```python
from build123d import *

# Parameters (mm, degrees)
F1_W     = 25.4
F1_H     = 12.7
F2_DEPTH = 25.4
F0_W     = 38.1
F0_H     = 50.8
F3_DEPTH = 12.7
F4_R     = 10.3422808599
F5_DEPTH = 12.701
F6_R     = 19.04999
F7_W     = 12.7
F7_H     = 6.35
F8_DEPTH = 12.7


# Not quite as in the source:
# - a fillet or chamfer is up to 0.001 mm smaller than in the source, because OpenCascade refuses the exact size


with BuildPart() as f2:
    # F1 (on face) → F2 (new body)
    with BuildSketch(Plane.XY):
        with Locations((6.35, 19.05)):
            Rectangle(F1_W, F1_H)
    extrude(amount=F2_DEPTH)

    # F0 (on Top) → F3 (join)
    with BuildSketch(Plane.XY):
        Rectangle(F0_W, F0_H)
    extrude(amount=F3_DEPTH)

    # F4 (on face) → F5 (cut, through all)
    with BuildSketch(Plane.XY.offset(12.7)):
        with Locations((0, -6.35)):
            Circle(F4_R)
    extrude(amount=-F5_DEPTH, mode=Mode.SUBTRACT)

    # F6 (radius 19.05 in the source; OpenCascade refuses exactly that, so slightly less here)
    f6_edges = [f2.edges().sort_by_distance(p)[0] for p in [
        (-19.05, -25.4, 6.35),
        (19.05, -25.4, 6.35),
    ]]
    fillet(f6_edges, radius=F6_R)

    # F7 (on face) → F8 (join)
    with BuildSketch(Plane(origin=(-6.35, 0, 0), x_dir=(0, -1, 0), z_dir=(-1, 0, 0))):
        with Locations((-19.05, 15.875)):
            Rectangle(F7_W, F7_H)
    extrude(amount=F8_DEPTH)


solid = f2.part
```
Geometry check sheet. Reference: the model listing, model coordinates, mm. A direction names the side the tool comes from. Coordinates: 2 decimals unless noted, no trailing zeros. Loops run counter-clockwise (first coordinate to the right, second up) from the corner with the lowest first, then second, coordinate; pieces in that order, holes last.
Item 1: Sectioned sample at D-D, the plane x = 16. Record the boundary of the cut face in (y, z), then the cut area to 3 significant figures.
Item 2: Release check for a two-part mould opening along X. For faces 4 (the face through (-2.242, -16.446, 6.439)), 5 (the face through (8, 2, 12.7)), 6 (the face through (19.05, 13, 10)) record: released by +X, released by -X, zero draft, split by the parting line, or undercut.
Item 3: Thickness scan on line 1 (Y direction, x = 0, z = 6.5); line 2 (Z direction, x = 14, y = 4); line 3 (Y direction, x = -13, z = 14.5). Record the ranges inside material, lowest first.
Item 4: Sectioned sample at C-C, the plane y = 7. Record the boundary of the cut face in (x, z).
Item 5: Go/stop test with flat-tipped pins: pin 1 Ø1.5 at (x, y) = (-0.5, -18.5) entering from +Z; pin 2 Ø18.5 at (x, y) = (0, -6.35) entering from -Z; pin 3 Ø4 at (x, z) = (8.5, 9.5) entering from -Y; pin 4 Ø10 at (x, y) = (-15, 19.5) entering from +Z. Record where each tip stops, or that it passes through.
Item 6: Access from +Z, -Z, +X, -X, +Y, -Y to the whole of each face (thin tool, end or side, straight path). Record for faces 1 (the face through (-6.35, 19, 22)), 2 (the face through (5, 12.7, 19)), 3 (the face through (13.32, -19.97, 6.44)).
Item 7: Sectioned sample at B-B, the plane y = -2. Record the boundary of the cut face in (x, z), then the cut area to 3 significant figures.
Check result:
1. outline: (-16.69, 0) - (25.4, 0) - (25.4, 25.4) - (12.7, 25.4) - (12.7, 12.7) - (-16.69, 12.7) - close
1. area: 696 mm2
2. face 4: undercut
2. face 5: zero draft
2. face 6: released by +X
3. line 1: y = -25.4 to -16.69, 3.99 to 25.4
3. line 2: z = 0 to 12.7
3. line 3: y = 12.7 to 25.4
4. outline: (-19.05, 0) - (19.05, 0) - (19.05, 12.7) - (-19.05, 12.7) - close
5. pin 1: stops at z = 12.7
5. pin 2: passes through
5. pin 3: stops at y = -24.26
5. pin 4: stops at z = 19.05
6. face 1: +Z, -X, +Y, -Y
6. face 2: +Z, +X, -X, -Y
6. face 3: +Z, -Z, +X, -Y
7. outline: (-19.05, 0) - (-9.38, 0) - (-9.38, 12.7) - (-19.05, 12.7) - close; (9.38, 0) - (19.05, 0) - (19.05, 12.7) - (9.38, 12.7) - close
7. area: 246 mm2
